Check sheet for the drawn part. Datum: minimum x, y, z corner. Units: mm. Give positions to 0.01 mm unless a question says otherwise; leave off trailing zeros. Write each loop counter-clockwise with the first axis right and the second up, starting at its lowest first coordinate (ties: lowest second). Pieces come first, ordered by that corner, then holes. Notation, with made-up numbers: M -11,42.25 L 33,42.25 A16 ccw 33,59.25 Z; hole C 12,24 d4. An arc over 180 degrees is marked long. Write item = value, one per line. Start each with the question number.
1) Gauge pin test, flat ends, axial feed: pin 1 (2 mm diameter, centred on x = 73.5, y = 5, fed in from -Z); pin 2 (5 mm diameter, centred on y = 7, z = 46, fed in from -X) (3 decimals); pin 3 (5 mm diameter, centred on y = 6.5, z = 95, fed in from +X) (3 decimals). Record the tip position at first contact, or that the pin passes through.
2) Sectioned sample at B-B, the plane x = 90. Record the cut outline in (y, z) (3 decimals).
3) Scan lines: L1, parallel to X at y = 5, z = 138 (3 decimals); L2, parallel to Z at x = 104, y = 8 (3 decimals); L3, parallel to X at y = 8.5, z = 110.5 (3 decimals). Record each from-to range of solid material in increasing order.
4) Sectioned sample at A-A, the plane z = 46. Record the cut outline in (x, y) (3 decimals), then the cut area to 3 significant figures.
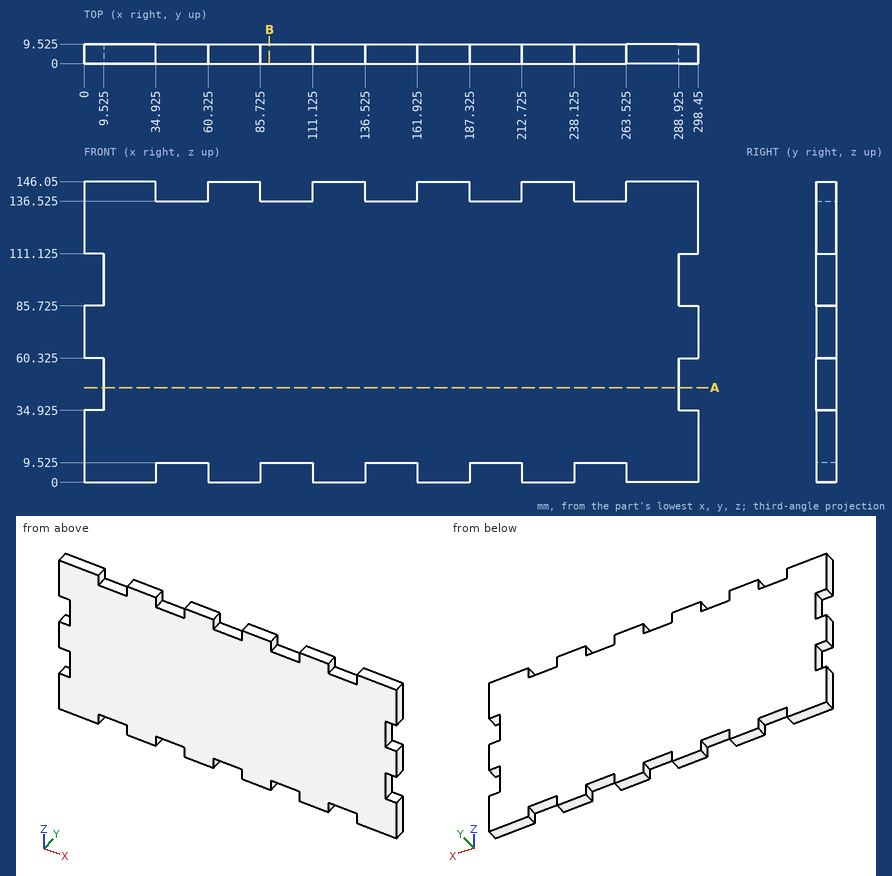
Data:
q1.pin_1 = 0
q1.pin_2 = 9.525
q1.pin_3 = 288.925
q2.outline = M 0,9.525 L 9.525,9.525 L 9.525,136.525 L 0,136.525 Z
q3.L1 = 0 to 34.925, 60.325 to 85.725, 111.125 to 136.525, 161.925 to 187.325, 212.725 to 238.125, 263.525 to 298.45
q3.L2 = 9.525 to 136.525
q3.L3 = 9.525 to 288.925
q4.outline = M 9.525,0 L 288.925,0 L 288.925,9.525 L 9.525,9.525 Z
q4.area = 2,660 mm2
